Verification items for the finished model (mm, model axes). Face numbers are marked on the shaded views. A direction names the side the tool comes from. Give positions to 0.01 mm unless a question says otherwise; leave off trailing zeros. Order: outer loops, then holes, each group sorted by start corner. A loop starts at its lowest first (then second) coordinate and runs counter-clockwise, first axis right, second up.
from build123d import *

# Parameters (mm, degrees)
F0_W     = 48.26
F0_H     = 45.72
F1_DEPTH = 9.398
F2_W     = 28.956
F2_H     = 33.02
F3_DEPTH = 25.4
F4_W     = 10.922
F4_H     = 41.275
F5_DEPTH = 2.794
F7_DEPTH = 6.605
F8_R     = 5.08
F9_R     = 1.5875
F10_R    = 5.08


with BuildPart() as f1:
    # F0 (on Top) → F1 (new body)
    with BuildSketch(Plane.XY):
        with Locations((24.13, 22.86)):
            Rectangle(F0_W, F0_H)
    extrude(amount=F1_DEPTH)

    # F2 (on face) → F3 (cut)
    with BuildSketch(Plane.XY.offset(9.398)):
        with Locations((33.782, 29.21)):
            Rectangle(F2_W, F2_H)
    extrude(amount=-F3_DEPTH, mode=Mode.SUBTRACT)

    # F4 (on face) → F5 (cut)
    with BuildSketch(Plane.XY.offset(9.398)):
        with Locations((9.652, 22.86)):
            Rectangle(F4_W, F4_H)
    extrude(amount=-F5_DEPTH, mode=Mode.SUBTRACT)

    # F6 (on face) → F7 (cut, through all)
    with BuildSketch(Plane.XY.offset(6.604)):
        with BuildLine():
            ThreePointArc((12.573, 36.449), (9.652, 39.37), (6.731, 36.449))
            Line((6.731, 36.449), (6.731, 8.509))
            ThreePointArc((6.731, 8.509), (9.652, 5.588), (12.573, 8.509))
            Line((12.573, 8.509), (12.573, 36.449))
        make_face()
    extrude(amount=-F7_DEPTH, mode=Mode.SUBTRACT)

    # F8
    f8_edges = [f1.edges().sort_by_distance(p)[0] for p in [
        (19.304, 12.7, 4.699),
    ]]
    fillet(f8_edges, radius=F8_R)

    # F9
    f9_edges = [f1.edges().sort_by_distance(p)[0] for p in [
        (4.191, 43.4975, 8.001),
        (4.191, 2.2225, 8.001),
        (15.113, 2.2225, 8.001),
        (15.113, 43.4975, 8.001),
    ]]
    fillet(f9_edges, radius=F9_R)

    # F10
    f10_edges = [f1.edges().sort_by_distance(p)[0] for p in [
        (48.26, 0, 4.699),
        (48.26, 12.7, 4.699),
    ]]
    fillet(f10_edges, radius=F10_R)


solid = f1.part
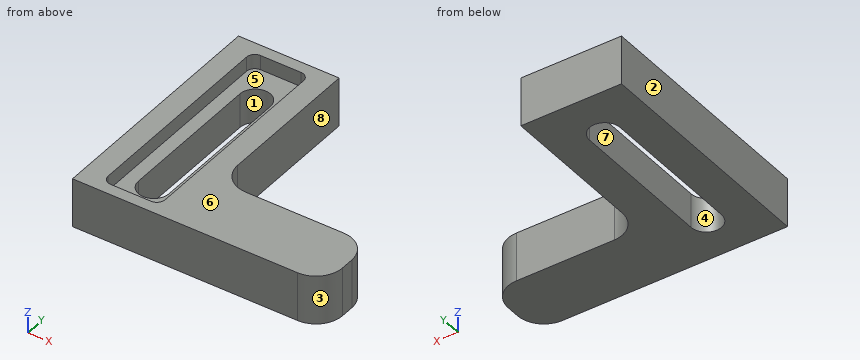
(1) Scan lines: line 1 (X direction, y = 28, z = 2.25); line 2 (X direction, y = 38.5, z = 8.75); line 3 (Y direction, x = 37, z = 1.75). Record each from-to range of solid material in increasing order.
Solved:
line 1: x = 0 to 6.73, 12.57 to 19.3
line 2: x = 0 to 4.19, 15.11 to 19.3
line 3: y = 0 to 12.7
(2) Set-up check for the marked faces 5, 6, 7 and 8: record each of +Z, -Z, +X, -X, +Y, -Y from which the full face is reachable in a straight line by a thin tool's end or side.
Solved:
face 5: +Z
face 6: +Z, +X, -X, +Y, -Y
face 7: +Z, -Z
face 8: +Z, -Z, +X, +Y
(3) Section check A-A, the plane y = 26.5. Enter the section's corners in (x, z).
Solved:
outline: (0, 0) - (6.73, 0) - (6.73, 6.6) - (4.19, 6.6) - (4.19, 9.4) - (0, 9.4) - close; (12.57, 0) - (19.3, 0) - (19.3, 9.4) - (15.11, 9.4) - (15.11, 6.6) - (12.57, 6.6) - close
(4) Release check for a two-part mould opening along Y. For the marked faces 1, 2, 3 and 4 record: pulls with the +Y half, pulls with the -Y half, needs draft (parallel to the pull), parting line crosses it, or undercut.
Solved:
face 1: undercut
face 2: needs draft
face 3: pulls with the -Y half
face 4: undercut
(5) Go/stop test with a flat-tipped pin: pin 1 (2 mm diameter, centred on y = 21.5, z = 2.5, fed in from +X). Record where the tip stops, or that it passes through.
Solved:
pin 1: stops at x = 19.3
(6) Section check D-D, the plane y = 40.5. Enter the section's corners in (x, z), then the cut area to 3 significant figures.
Solved:
outline: (0, 0) - (19.3, 0) - (19.3, 9.4) - (15.11, 9.4) - (15.11, 6.6) - (4.19, 6.6) - (4.19, 9.4) - (0, 9.4) - close
area: 151 mm2
(7) Section check C-C, the plane x = 11.5. Enter the section's corners in (y, z).
Solved:
outline: (0, 0) - (6.25, 0) - (6.25, 6.6) - (2.22, 6.6) - (2.22, 9.4) - (0, 9.4) - close; (38.71, 0) - (45.72, 0) - (45.72, 9.4) - (43.5, 9.4) - (43.5, 6.6) - (38.71, 6.6) - close
(8) Section check B-B, the plane z = 8. Enter the section's corners in (x, y) (1 decimal), then the cut area to 3 significant figures.
Solved:
outline: (0, 0) - (43.2, 0) arc R5.1 ccw to (48.3, 5.1) - (48.3, 7.6) arc R5.1 ccw to (43.2, 12.7) - (24.4, 12.7) arc R5.1 cw to (19.3, 17.8) - (19.3, 45.7) - (0, 45.7) - close; hole (4.2, 3.8) arc R1.6 ccw to (5.8, 2.2) - (13.5, 2.2) arc R1.6 ccw to (15.1, 3.8) - (15.1, 41.9) arc R1.6 ccw to (13.5, 43.5) - (5.8, 43.5) arc R1.6 ccw to (4.2, 41.9) - close
area: 796 mm2
